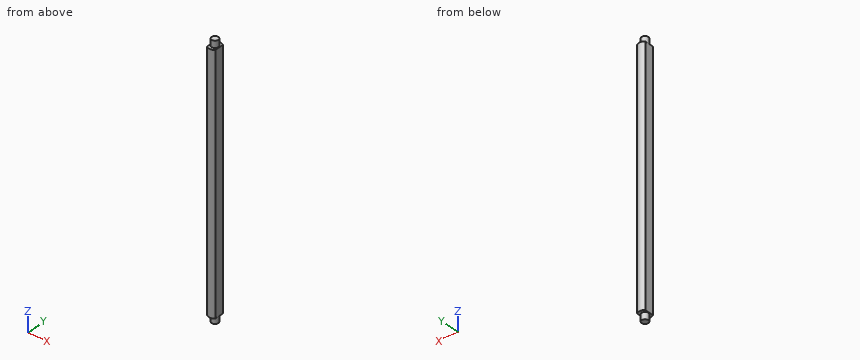
```python
from build123d import *

# Parameters (mm, degrees)
Y_KSEKLIK_EKSTR_ZYON1_DEPTH = 110
IZIM5_R                     = 1.5
Y_KSEKLIK_EKSTR_ZYON3_DEPTH = 3
Y_KSEKLIK_EKSTR_ZYON4_START = 3
IZIM6_R                     = 1.5
Y_KSEKLIK_EKSTR_ZYON4_DEPTH = 3


with BuildPart() as part:
    # Çizim2 → Yükseklik-Ekstrüzyon1 (new body)
    with BuildSketch(Plane.XY):
        with BuildLine():
            ThreePointArc((1.79891634, 2.08), (0, 2.75), (-1.79891634, 2.08))
            Line((-1.79891634, 2.08), (-1.79891634, -2.08))
            ThreePointArc((-1.79891634, -2.08), (0, -2.75), (1.79891634, -2.08))
            Line((1.79891634, -2.08), (1.79891634, 2.08))
        make_face()
    extrude(amount=Y_KSEKLIK_EKSTR_ZYON1_DEPTH)

    # Çizim5 → Yükseklik-Ekstrüzyon3 (add)
    with BuildSketch(Plane.XY.offset(110)):
        Circle(IZIM5_R)
    extrude(amount=Y_KSEKLIK_EKSTR_ZYON3_DEPTH)

    # Çizim6 → Yükseklik-Ekstrüzyon4 (add)
    with BuildSketch(Plane(origin=(0, 0, 0), x_dir=(-1, 0, 0), z_dir=(0, 0, -1)).offset(Y_KSEKLIK_EKSTR_ZYON4_START)):
        with Locations(Location((0, 0, 0), (0, 0, 180))):
            Circle(IZIM6_R)
    extrude(amount=-Y_KSEKLIK_EKSTR_ZYON4_DEPTH)


solid = part.part
```
For this review, take the finished solid that the model builds, in its own axes (mm). Round coordinates to 2 decimals unless told otherwise and drop trailing zeros. Write each loop counter-clockwise with the first axis right and the second up, starting at its lowest first coordinate (ties: lowest second). Pieces come first, ordered by that corner, then holes. Notation, with made-up numbers: M -6,-15 L 27,-15 A34 cw 27,20 Z; hole C -16.75,4 d3. An arc over 180 degrees is marked long. One line per item, written item: value. Start each with the question number.
(1) Wall thickness on line 1 (Z direction, x = 0.1, y = 1.55); line 2 (X direction, y = 2.1, z = 106); line 3 (Y direction, x = 0.3, z = 37): over which ranges is each line inside the solid? List them lowest first.
(2) We need section A-A (x = 0). Give the boundary of the cut face in (y, z).
(3) We need section B-B (z = 48). Give the boundary of the cut face in (x, y), and give its area (3 significant figures).
(4) Insertion check: pin 1 (1 mm diameter, centred on x = 1, z = 60, fed in from -Y). The pin has a flat end and moves straight along its axis. Give the tip position at first contact, or say it passes through.
Result:
1. line 1: 0 to 110
1. line 2: -1.78 to 1.78
1. line 3: -2.73 to 2.73
2. outline: M -2.75,0 L -1.5,0 L -1.5,-3 L 1.5,-3 L 1.5,0 L 2.75,0 L 2.75,110 L 1.5,110 L 1.5,113 L -1.5,113 L -1.5,110 L -2.75,110 Z
3. outline: M -1.8,-2.08 A2.75 ccw 1.8,-2.08 L 1.8,2.08 A2.75 ccw -1.8,2.08 Z
3. area: 18.3 mm²
4. pin 1: y = -2.7
